Part model, mm, in its own coordinate system. A direction names the side the tool comes from. Round coordinates to 2 decimals unless told otherwise and drop trailing zeros. Write each loop counter-clockwise with the first axis right and the second up, starting at its lowest first coordinate (ties: lowest second). Pieces come first, ordered by that corner, then holes. Notation, with made-up numbers: M 32,41.5 L 49,41.5 A20 ccw 49,49.5 Z; hole C -1.5,73.5 d9. An arc over 180 degrees is marked long. Use one line per item in the form item = value. Start each with the question number.
Item 1: Cut at D-D, the plane x = 15.5. Give the cut face in (y, z).
Item 2: Which spindle directions (+Z, -Z, +X, -X, +Y, -Y) get a long thin tool onto all of the face, cutting with end or side? Do faces 1 (the face through (1.7, -22.1, 0)), 2 (the face through (-1.5, -11.4, 10.7)), 3 (the face through (8.767, -16.856, 22.958)). Say none if no direction does.
Item 3: Probe L1, parallel to Y at x = 0, z = 6; L2, parallel to Z at x = -12, y = -21.5; L3, parallel to X at y = 5, z = 21. List the from-to ranges inside material, lowest first.
Item 4: Cut at A-A, the plane y = 0. Give the cut face in (x, z), then the cut area to 3 significant figures.
Item 5: Cut at C-C, the plane z = 23.5. Give the cut face in (x, y), then the cut area to 3 significant figures.
Item 6: Flat gauge pins, fed straight in: pin 1 Ø1.5 at (x, z) = (19.5, 8) entering from +Y; pin 2 Ø8 at (y, z) = (-15.5, 21.5) entering from +X; pin 3 Ø1.5 at (y, z) = (-2, 19) entering from +X. Where does each tip first touch, or does it go through?
from build123d import *

# Parameters (mm, degrees)
SKETCH1_R           = 25
BOSS_EXTRUDE1_DEPTH = 20
SKETCH2_R           = 19
BOSS_EXTRUDE2_DEPTH = 6
SKETCH3_R           = 11.5
CUT_EXTRUDE1_DEPTH  = 60
SKETCH5_R           = 22
SKETCH5_R_2         = 11.5
BOSS_EXTRUDE4_DEPTH = 5


with BuildPart() as part:
    # Sketch1 → Boss-Extrude1 (new body)
    with BuildSketch(Plane.XY):
        Circle(SKETCH1_R)
    extrude(amount=BOSS_EXTRUDE1_DEPTH)

    # Sketch2 → Boss-Extrude2 (add)
    with BuildSketch(Plane.XY.offset(20)):
        Circle(SKETCH2_R)
    extrude(amount=BOSS_EXTRUDE2_DEPTH)

    # Sketch3 → Cut-Extrude1 (cut)
    with BuildSketch(Plane.XY.offset(26)):
        Circle(SKETCH3_R)
    extrude(amount=-CUT_EXTRUDE1_DEPTH, mode=Mode.SUBTRACT)

    # Sketch5 → Boss-Extrude4 (add)
    with BuildSketch(Plane(origin=(0, 0, 0), x_dir=(-1, 0, 0), z_dir=(0, 0, -1))):
        Circle(SKETCH5_R)
        with Locations(Location((0, 0, 0), (0, 0, 180))):
            Circle(SKETCH5_R_2, mode=Mode.SUBTRACT)
    extrude(amount=BOSS_EXTRUDE4_DEPTH)


solid = part.part
Model answer:
q1.outline = M -19.62,0 L -15.61,0 L -15.61,-5 L 15.61,-5 L 15.61,0 L 19.62,0 L 19.62,20 L 10.99,20 L 10.99,26 L -10.99,26 L -10.99,20 L -19.62,20 Z
q2.face_1 = -Z
q2.face_2 = +Z, -Z
q2.face_3 = +Z
q3.L1 = -25 to -11.5, 11.5 to 25
q3.L2 = 0 to 20
q3.L3 = -18.33 to -10.36, 10.36 to 18.33
q4.outline = M -25,0 L -22,0 L -22,-5 L -11.5,-5 L -11.5,26 L -19,26 L -19,20 L -25,20 Z; M 11.5,-5 L 22,-5 L 22,0 L 25,0 L 25,20 L 19,20 L 19,26 L 11.5,26 Z
q4.area = 735 mm²
q5.outline = C 0,0 d38; hole C 0,0 d23
q5.area = 719 mm²
q6.pin_1 = 16.54
q6.pin_2 = 22.04
q6.pin_3 = 24.97
